Could you check a few things on this model? Use its own coordinates, in mm. A direction names the side the tool comes from. Give positions to 0.01 mm unless a question says otherwise; leave off trailing zeros. Write each loop counter-clockwise with the first axis right and the second up, starting at its lowest first coordinate (ties: lowest second). Pieces come first, ordered by that corner, then holes. Notation, with made-up numbers: (1.25, -32) - (19.25, -32) arc R23 cw to (19.25, -9) - close; hole circle Ø7 at (-21, -4.75). An arc over 180 degrees is marked (long way). Answer as CSV lines item,"result". Start each with the question number.
Q1. On a 3-axis mill with a long thin cutter (end or side, diameter ignored), from which of +Z, -Z, +X, -X, +Y, -Y can I reach the whole of each face in a straight line? I mean faces 4 (the face through (0.69, -3.1, -43.32)), 5 (the face through (-56.934, 17.929, 46.975)). Say none if no direction works.
Q2. We'd pull the mould along Y, two halves only. Please class faces 1 (the face through (10.327, -46.507, -11.144)), 2 (the face through (42, 43, 56.399)), 3 (the face through (-47.056, -19.51, -13.676)): pulls with the +Y half, pulls with the -Y half, needs draft (parallel to the pull), parting line crosses it, or undercut.
Q3. Will these pins go through, and if not, where does the flat tip stop? pin 1 Ø2 at (x, z) = (-11.5, 39.5) entering from -Y; pin 2 Ø10 at (x, z) = (-6.5, 24.5) entering from +Y; pin 3 Ø2 at (x, z) = (38.5, 41.5) entering from -Y.
Q4. Imagine slicing it at C-C on z = -36. List the corners of the cut face in (x, y) for me.
Q5. Imagine slicing it at A-A on y = 0. List the corners of the cut face in (x, z) for me (3 decimals), and give its area (3 significant figures).
Q6. If I drill on line 1 along Z through (x, y) = (-9, -37.5); line 2 along Y through (x, z) = (-37.5, 38); line 3 along X through (y, z) = (-3.5, 5), over which ranges is the centre line in solid material (lowest first)?
```python
from build123d import *

# Parameters (mm, degrees)
F2_T = -3.81
F4_D = 6.35


with BuildPart() as f1:
    # F0 (on Front) → F1 (revolve)
    with BuildSketch(Plane.XZ):
        Polygon((0, -45.200619), (0, 56.399381), (-63.5, 56.399381), (-63.5, 37.349381), (-43.18, -45.200619), align=None)
    revolve(axis=Axis((0, 0, 6.864863), (0, 0, -1)))

    # F2
    f2_openings = [f1.faces().sort_by_distance(p)[0] for p in [
        (0, 0, 56.399381),
    ]]
    offset(amount=F2_T, openings=f2_openings)

    # F4 (through all)
    with Locations(Plane.XY.offset(-41.390619)):
        with Locations((0, 0)):
            Hole(F4_D / 2)


solid = f1.part
```
Conclusion:
1,face 4,"+Z, -Z"
1,face 5,"+Z"
2,face 1,"undercut"
2,face 2,"needs draft"
2,face 3,"parting line crosses it"
3,pin 1,"y = -62.63"
3,pin 2,"y = 61.31"
3,pin 3,"y = -51.24"
4,outline,"circle Ø90.89 at (0, 0); hole circle Ø83.04 at (0, 0)"
5,outline,"(-63.5, 37.349) - (-43.18, -45.201) - (-3.175, -45.201) - (-3.175, -41.391) - (-40.194, -41.391) - (-59.69, 37.811) - (-59.69, 56.399) - (-63.5, 56.399) - close; (3.175, -45.201) - (43.18, -45.201) - (63.5, 37.349) - (63.5, 56.399) - (59.69, 56.399) - (59.69, 37.811) - (40.194, -41.391) - (3.175, -41.391) - close"
5,area,"1,070 mm^2"
6,line 1,"-45.2 to -41.39"
6,line 2,"-51.24 to -46.44, 46.44 to 51.24"
6,line 3,"-55.43 to -51.49, 51.49 to 55.43"
